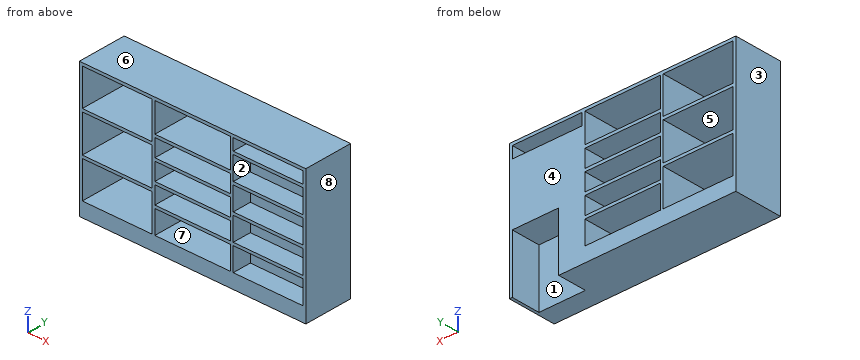
```python
from build123d import *

# Parameters (mm, degrees)
F0_W     = 1950
F0_H     = 1150
F1_DEPTH = 420
F2_W     = 650
F2_H     = 200
F2_H_2   = 150
F2_H_3   = 250
F2_W_2   = 600
F2_H_4   = 315
F2_H_5   = 320
F3_DEPTH = 450
F4_W     = 600
F4_H     = 200
F5_DEPTH = 160
F6_W     = 600
F6_H     = 100
F7_DEPTH = 450
F8_W     = 400
F8_H     = 250
F9_DEPTH = 500


with BuildPart() as f1:
    # F0 (on Front) → F1 (new body)
    with BuildSketch(Plane.XZ):
        with Locations((934.696341, 542.311319)):
            Rectangle(F0_W, F0_H)
    extrude(amount=F1_DEPTH)

    # F2 (on face) → F3 (cut)
    with BuildSketch(Plane.XZ.offset(420)):
        with Locations((934.696341, 192.311319)):
            Rectangle(F2_W, F2_H)
        with Locations((934.696341, 392.311319)):
            Rectangle(F2_W, F2_H_2)
        with Locations((934.696341, 567.311319)):
            Rectangle(F2_W, F2_H_2)
        with Locations((934.696341, 742.311319)):
            Rectangle(F2_W, F2_H_2)
        with Locations((934.696341, 967.311319)):
            Rectangle(F2_W, F2_H_3)
        with Locations((284.696341, 934.811319)):
            Rectangle(F2_W_2, F2_H_4)
        with Locations((284.696341, 592.311319)):
            Rectangle(F2_W_2, F2_H_5)
        with Locations((284.696341, 249.811319)):
            Rectangle(F2_W_2, F2_H_4)
    extrude(amount=-F3_DEPTH, mode=Mode.SUBTRACT)

    # F4 (on face) → F5 (cut)
    with BuildSketch(Plane.XZ.offset(420)):
        Polygon((1884.696341, 967.311319), (1284.696341, 967.311319), (1284.696341, 842.311319), (1284.696341, 817.311319), (1284.696341, 767.311319), (1884.696341, 767.311319), (1884.696341, 817.311319), (1884.696341, 842.311319), align=None)
        with Locations((1584.696341, 642.311319)):
            Rectangle(F4_W, F4_H)
        with Locations((1584.696341, 417.311319)):
            Rectangle(F4_W, F4_H)
        with Locations((1584.696341, 192.311319)):
            Rectangle(F4_W, F4_H)
    extrude(amount=-F5_DEPTH, mode=Mode.SUBTRACT)

    # F6 (on face) → F7 (cut)
    with BuildSketch(Plane.XZ.offset(420)):
        with Locations((1584.696341, 1042.311319)):
            Rectangle(F6_W, F6_H)
    extrude(amount=-F7_DEPTH, mode=Mode.SUBTRACT)

    # F8 (on face) → F9 (cut)
    with BuildSketch(Plane(origin=(0, 0, -32.688681), x_dir=(1, 0, 0), z_dir=(0, 0, -1))):
        with Locations((1684.696341, 125)):
            Rectangle(F8_W, F8_H)
    extrude(amount=-F9_DEPTH, mode=Mode.SUBTRACT)


solid = f1.part
```
CAD build for the part. Positions are in the model's coordinates, mm. Face numbers are marked on the shaded views. A direction names the side the tool comes from. Round coordinates to 2 decimals unless told otherwise and drop trailing zeros. Loops run counter-clockwise (first coordinate to the right, second up) from the corner with the lowest first, then second, coordinate; pieces in that order, holes last. Notation, with made-up numbers: M 33,87 L 81,87 A13 ccw 81,100 Z; hole C -33.75,82.5 d7. An arc over 180 degrees is marked long. Use a Markdown table: item, result. Add a question column.
(1) Cut at C-C (z = 72). Give the cut face in (x, y), and give its area (3 significant figures).
(2) Which spindle directions (+Z, -Z, +X, -X, +Y, -Y) get a long thin tool onto all of the face, cutting with end or side? Do the marked faces 1, 2, 3, 4 and 5. Say none if no direction does.
(3) Cut at D-D (z = 910). Give the cut face in (x, y).
(4) Cut at A-A (x = 1681). Give the cut face in (y, z), and give its area (3 significant figures).
(5) Cut at B-B (x = 133.5). Give the cut face in (y, z), and give its area (3 significant figures).
(6) Pull direction X, two halves, no side cores. Call the marked faces 6, 7 and 8: +X half, -X half, draft (parallel to the pull), parting line (faces both ways), or undercut.
(7) Drill centre lines: line 1 (Z direction, x = 531, y = -337.5); line 2 (Z direction, x = 1158.5, y = -91.5); line 3 (X direction, y = -340, z = 183). Where is each one in solid material? Low to high.
Geometry says:
| question | item | result |
|---|---|---|
| 1 | outline | M -40.3,-420 L 1909.7,-420 L 1909.7,0 L 1884.7,0 L 1884.7,-250 L 1484.7,-250 L 1484.7,0 L -40.3,0 Z |
| 1 | area | 719,000 mm² |
| 2 | face 1 | -Z, +Y |
| 2 | face 2 | -Y |
| 2 | face 3 | +Z, -Z, -X, +Y, -Y |
| 2 | face 4 | +Z, -Z, +X, -X, +Y |
| 2 | face 5 | +Y, -Y |
| 3 | outline | M -40.3,-420 L -15.3,-420 L -15.3,0 L -40.3,0 Z; M 584.7,-420 L 609.7,-420 L 609.7,0 L 584.7,0 Z; M 1259.7,-420 L 1284.7,-420 L 1284.7,-260 L 1884.7,-260 L 1884.7,-420 L 1909.7,-420 L 1909.7,0 L 1259.7,0 Z |
| 4 | outline | M -420,-32.69 L -250,-32.69 L -250,467.31 L 0,467.31 L 0,992.31 L -420,992.31 L -420,967.31 L -260,967.31 L -260,767.31 L -420,767.31 L -420,742.31 L -260,742.31 L -260,542.31 L -420,542.31 L -420,517.31 L -260,517.31 L -260,317.31 L -420,317.31 L -420,292.31 L -260,292.31 L -260,92.31 L -420,92.31 Z; M -420,1092.31 L 0,1092.31 L 0,1117.31 L -420,1117.31 Z |
| 4 | area | 188,000 mm² |
| 5 | outline | M -420,-32.69 L 0,-32.69 L 0,92.31 L -420,92.31 Z; M -420,407.31 L 0,407.31 L 0,432.31 L -420,432.31 Z; M -420,752.31 L 0,752.31 L 0,777.31 L -420,777.31 Z; M -420,1092.31 L 0,1092.31 L 0,1117.31 L -420,1117.31 Z |
| 5 | area | 84,000 mm² |
| 6 | face 6 | draft |
| 6 | face 7 | undercut |
| 6 | face 8 | +X half |
| 7 | line 1 | z = -32.69 to 92.31, 407.31 to 432.31, 752.31 to 777.31, 1092.31 to 1117.31 |
| 7 | line 2 | z = -32.69 to 92.31, 292.31 to 317.31, 467.31 to 492.31, 642.31 to 667.31, 817.31 to 842.31, 1092.31 to 1117.31 |
| 7 | line 3 | x = -40.3 to -15.3, 584.7 to 609.7, 1259.7 to 1284.7, 1884.7 to 1909.7 |
